Input: part model. Units: mm. Frame: model coordinates. Face numbers are marked on the shaded views. Give positions to 0.01 mm unless a question says otherwise; leave off trailing zeros. Loops run counter-clockwise (first coordinate to the right, second up) from the corner with the lowest first, then second, coordinate; pieces in that order, holes last. Notation, with made-up numbers: (18.25, -32.5) -> (22.25, -32.5) arc R18 cw to (22.25, -8.5) -> close; hole circle Ø5 at (30.5, 88.25). An arc over 180 degrees is marked (long way). One line per question, with ' | ' between items.
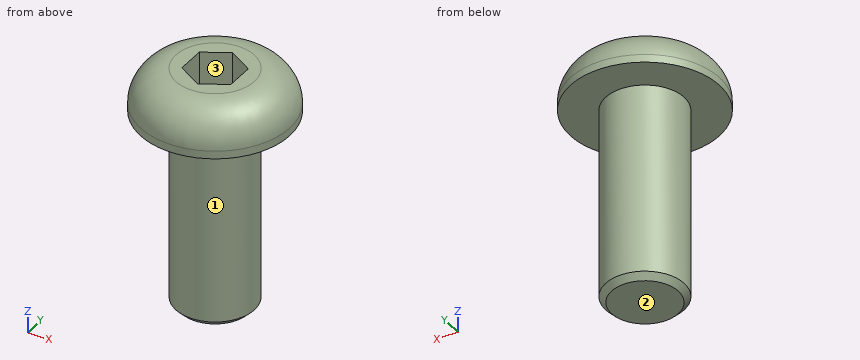
from build123d import *

# Parameters (mm, degrees)
SKETCH1_R           = 3.8
BOSS_EXTRUDE1_DEPTH = 2.2
SKETCH2_R           = 2
BOSS_EXTRUDE2_DEPTH = 10
CHAMFER1_SIZE       = 0.3
CUT_EXTRUDE1_DEPTH  = 2
FILLET1_R           = 1.8


with BuildPart() as part:
    # Sketch1 → Boss-Extrude1 (new body)
    with BuildSketch(Plane.XY):
        Circle(SKETCH1_R)
    extrude(amount=BOSS_EXTRUDE1_DEPTH)

    # Sketch2 → Boss-Extrude2 (add)
    with BuildSketch(Plane(origin=(0, 0, 0), x_dir=(-1, 0, 0), z_dir=(0, 0, -1))):
        Circle(SKETCH2_R)
    extrude(amount=BOSS_EXTRUDE2_DEPTH)

    # Chamfer1
    chamfer1_edges = [part.edges().sort_by_distance(p)[0] for p in [
        (2, 0, -10),
    ]]
    chamfer(chamfer1_edges, length=CHAMFER1_SIZE)

    # Sketch3 → Cut-Extrude1 (cut)
    with BuildSketch(Plane.XY.offset(2.2)):
        Polygon((0, 1.443375673), (-1.25, 0.721687836), (-1.25, -0.721687836), (0, -1.443375673), (1.25, -0.721687836), (1.25, 0.721687836), align=None)
    extrude(amount=-CUT_EXTRUDE1_DEPTH, mode=Mode.SUBTRACT)

    # Fillet1
    fillet1_edges = [part.edges().sort_by_distance(p)[0] for p in [
        (-3.8, 0, 2.2),
    ]]
    fillet(fillet1_edges, radius=FILLET1_R)


solid = part.part
1. Pull-direction query (X, two-part tool) for the marked faces 1, 2 and 3; classes: pulls with the +X half, pulls with the -X half, needs draft (parallel to the pull), parting line crosses it, or undercut.
Determined:
face 1: parting line crosses it | face 2: needs draft | face 3: undercut
2. Ray query, line 1 along X through (y, z) = (0.75, 1); line 2 along Z through (x, y) = (0, 0.5); line 3 along Z through (x, y) = (3.25, 1.5). Return the intervals inside material, ascending. Write a range as from..to.
Determined:
line 1: x = -3.62..-1.2, 1.2..3.62 | line 2: z = -10..0.2 | line 3: z = 0..1.26
3. Section query B-B (z = -1.75). Output: boundary loops of the cut face in (x, y), then the cut area to 3 significant figures.
Determined:
outline: circle Ø4 at (0, 0) | area: 12.6 mm2
4. Section query A-A (y = 0). Output: boundary loops of the cut face in (x, z).
Determined:
outline: (-3.8, 0) -> (-2, 0) -> (-2, -9.7) -> (-1.7, -10) -> (1.7, -10) -> (2, -9.7) -> (2, 0) -> (3.8, 0) -> (3.8, 0.4) arc R1.8 ccw to (2, 2.2) -> (1.25, 2.2) -> (1.25, 0.2) -> (-1.25, 0.2) -> (-1.25, 2.2) -> (-2, 2.2) arc R1.8 ccw to (-3.8, 0.4) -> close
5. Pin query (flat end, axial travel): P1, Ø2, axis at x = -1.5, z = -5.5, coming from the +Y side; P2, Ø4, axis at x = -0.5, z = -5.5, coming from the +Y side; P3, Ø0.7, axis at y = -0.5, z = 1, coming from the -X side. Return the tip coordinate at first contact, or that it passes through.
Determined:
P1: stops at y = 1.94 | P2: stops at y = 2 | P3: stops at x = -3.76
